from build123d import *

# Parameters (mm, degrees)
SKETCH_1_R        = 20
SKETCH_1_R_2      = 18
EXTRUDE_1_DEPTH   = 24
EXTRUDE_1_2_DEPTH = 24
SKETCH_2_R        = 20
EXTRUDE_2_DEPTH   = 2


with BuildPart() as part:
    # Sketch 1 → Extrude 1 (new body)
    with BuildSketch(Plane.XY):
        Circle(SKETCH_1_R)
        Circle(SKETCH_1_R_2, mode=Mode.SUBTRACT)
    extrude(amount=EXTRUDE_1_DEPTH)



with BuildPart() as body_2:
    # Sketch 1 → Extrude 1 2 (new body)
    with BuildSketch(Plane.XY):
        Polygon((4.099186911, -7.1), (8.198373822, 0), (4.099186911, 7.1), (-4.099186911, 7.1), (-8.198373822, 0), (-4.099186911, -7.1), align=None)
        Polygon((2.944486373, -5.1), (5.888972746, 0), (2.944486373, 5.1), (-2.944486373, 5.1), (-5.888972746, 0), (-2.944486373, -5.1), align=None, mode=Mode.SUBTRACT)
    extrude(amount=EXTRUDE_1_2_DEPTH)


with BuildPart() as part_1:
    add(part.part)

    add(body_2.part)  # Extrude 2 merges body 2
    # Sketch 2 → Extrude 2 (add)
    with BuildSketch(Plane(origin=(0, 0, 0), x_dir=(-1, 0, 0), z_dir=(0, 0, -1))):
        with Locations(Location((0, 0, 0), (0, 0, 180))):
            Circle(SKETCH_2_R)
        Polygon((2.944486373, 5.1), (5.888972746, 0), (2.944486373, -5.1), (-2.944486373, -5.1), (-5.888972746, 0), (-2.944486373, 5.1), align=None, mode=Mode.SUBTRACT)
    extrude(amount=-EXTRUDE_2_DEPTH)


solid = part_1.part
Check sheet for the modelled part. Datum: model origin and axes. Units: mm. A direction names the side the tool comes from. Give positions to 0.01 mm unless a question says otherwise; leave off trailing zeros. Write each loop counter-clockwise with the first axis right and the second up, starting at its lowest first coordinate (ties: lowest second). Pieces come first, ordered by that corner, then holes. Notation, with made-up numbers: (46, -16) -> (76, -16) arc R11 ccw to (76, -3) -> close; hole circle Ø3 at (-0.5, -32.5). An arc over 180 degrees is marked (long way). Use one line per item in the form item = value. Start each with the question number.
1. Section check B-B (x = 0). Record the cut outline in (y, z).
2. Section check A-A (z = 17.5). Record the cut outline in (x, y), and give its area (3 significant figures).
3. Section check C-C (y = -4). Record the cut outline in (x, z), and give its area (3 significant figures).
4. Thickness scan on line 1 along Y through (x, z) = (0, 15.25); line 2 along X through (y, z) = (-4, 7); line 3 along Y through (x, z) = (1.5, 6.25). Record the ranges inside material, lowest first. Write a range as from..to.
5. Go/stop test with flat-tipped pins: P1, Ø3, axis at x = -13, z = 12.5, coming from the -Y side; P2, Ø4, axis at x = 1, z = 13, coming from the +Y side; P3, Ø6, axis at x = -7.5, y = 7.5, coming from the +Z side. Record where each tip stops, or that it passes through.
6. Access from +Z, -Z, +X, -X, +Y, -Y to the whole of each face (thin tool, end or side, straight path). Record for faces 4 (the flat face through (5, -2, 24)), 5 (the flat face through (-6.12, 3.6, 12.85)), 6 (the flat face through (-4.396, 2.586, 11.832)).
7. Section check D-D (y = 6). Record the cut outline in (x, z), and give its area (3 significant figures).
8. Mould release check, pull along X, two halves, no side actions. Record for faces 1 (the flat face through (4, -4, 0)), 2 (the flat face through (0, -7.1, 13)), 3 (the cylindrical face through (-4.336, -19.524, 11.832)): pulls with the +X half, pulls with the -X half, needs draft (parallel to the pull), parting line crosses it, or undercut.
Conclusion:
q1.outline = (-20, 0) -> (-5.1, 0) -> (-5.1, 24) -> (-7.1, 24) -> (-7.1, 2) -> (-18, 2) -> (-18, 24) -> (-20, 24) -> close; (5.1, 0) -> (20, 0) -> (20, 24) -> (18, 24) -> (18, 2) -> (7.1, 2) -> (7.1, 24) -> (5.1, 24) -> close
q2.outline = circle Ø40 at (0, 0); (-8.2, 0) -> (-4.1, -7.1) -> (4.1, -7.1) -> (8.2, 0) -> (4.1, 7.1) -> (-4.1, 7.1) -> close; hole circle Ø36 at (0, 0); hole (-5.89, 0) -> (-2.94, -5.1) -> (2.94, -5.1) -> (5.89, 0) -> (2.94, 5.1) -> (-2.94, 5.1) -> close
q2.area = 323 mm²
q3.outline = (-19.6, 0) -> (-3.58, 0) -> (-3.58, 24) -> (-5.89, 24) -> (-5.89, 2) -> (-17.55, 2) -> (-17.55, 24) -> (-19.6, 24) -> close; (3.58, 0) -> (19.6, 0) -> (19.6, 24) -> (17.55, 24) -> (17.55, 2) -> (5.89, 2) -> (5.89, 24) -> (3.58, 24) -> close
q3.area = 256 mm²
q4.line_1 = -20..-18, -7.1..-5.1, 5.1..7.1, 18..20
q4.line_2 = -19.6..-17.55, -5.89..-3.58, 3.58..5.89, 17.55..19.6
q4.line_3 = -19.94..-17.94, -7.1..-5.1, 5.1..7.1, 17.94..19.94
q5.P1 = -16.36
q5.P2 = 20
q5.P3 = 2
q6.face_4 = +Z, +X, -X, +Y, -Y
q6.face_5 = +Z
q6.face_6 = +Z, -Z
q7.outline = (-19.08, 0) -> (19.08, 0) -> (19.08, 24) -> (16.97, 24) -> (16.97, 2) -> (4.73, 2) -> (4.73, 24) -> (-4.73, 24) -> (-4.73, 2) -> (-16.97, 2) -> (-16.97, 24) -> (-19.08, 24) -> close
q7.area = 377 mm²
q8.face_1 = needs draft
q8.face_2 = undercut
q8.face_3 = parting line crosses it
